Design review of the part built by this model. Coordinates are the model's own, in mm. Face numbers are marked on the shaded views. Coordinates: 2 decimals unless noted, no trailing zeros. Order: outer loops, then holes, each group sorted by start corner. A loop starts at its lowest first (then second) coordinate and runs counter-clockwise, first axis right, second up. Notation, with made-up numbers: M 87.5,57.5 L 135.5,57.5 A16 cw 135.5,75.5 Z; hole C -8.75,4.5 d7. An arc over 180 degrees is marked long. Answer in a Markdown table with one row per item.
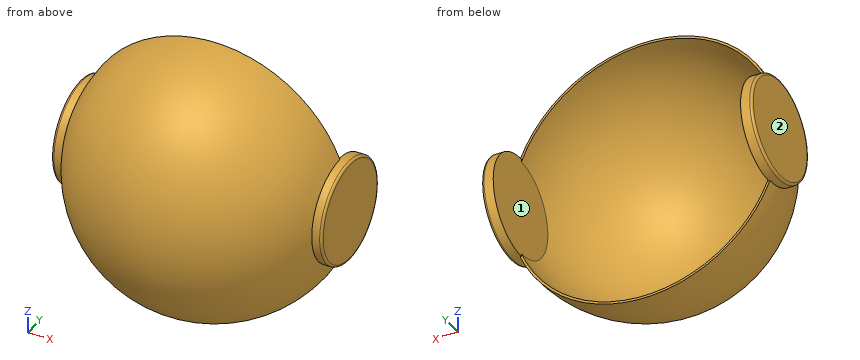
Autodesk Inventor part; units mm, degrees
ref_plane "Work Plane1" through (0, 0, 59) normal (0, 0, 1) x (1, 0, 0)
ref_plane "Work Plane2" through (-59, 0, 0) normal (1, 0, 0) x (0, 1, 0)
ref_plane "Work Plane3" through (59, 0, 0) normal (1, 0, 0) x (0, 1, 0)
sketch "Sketch1" plane through (0, 0, 0) normal (0, 0, 1) x (1, 0, 0)
  arc A0 (-59, 0) -> (59, 0) centre (0, 0) ccw
  arc A1 (-58, 0) -> (58, 0) centre (0, 0) ccw
  line L0 (-59, 0) -> (59, 0)
  dimension "d0" = 118
  dimension "d1" = 116
revolve "Revolution1" add sketch "Sketch1" angle 360 about axis through (-59, 0, 0) along (1, 0, 0) contours L0 A1 A0
ref_plane "Work Plane1" through (0, 0, 59) normal (0, 0, 1) x (1, 0, 0)
sketch "Sketch2" plane through (0, 0, 59) normal (0, 0, 1) x (1, 0, 0)
  circle A0 centre (0, 0) radius 59
  line L0 (-59, 0) -> (59, 0)
extrude "Extrusion1" cut sketch "Sketch2" against normal through all contours L0 A0 picked at (13.5288, 25.207)
ref_plane "Work Plane2" through (-59, 0, 0) normal (1, 0, 0) x (0, 1, 0)
sketch "Sketch3" plane through (-59, 0, 0) normal (1, 0, 0) x (0, 1, 0)
  circle A0 centre (0, 0) radius 22.5
  dimension "d5" = 45
extrude "Extrusion2" add sketch "Sketch3" along normal blind 5
fillet "Fillet1" radius 1 1 edges at (-59, -22.5, 0)
ref_plane "Work Plane3" through (59, 0, 0) normal (1, 0, 0) x (0, 1, 0)
sketch "Sketch4" plane through (59, 0, 0) normal (1, 0, 0) x (0, 1, 0)
  circle A0 centre (0, 0) radius 22.5
  point P0 (0, 22.5)
extrude "Extrusion3" add sketch "Sketch4" against normal blind 5
fillet "Fillet2" radius 1 1 edges at (59, -22.5, 0)
properties part number "Head"
(1) Draft analysis for pull direction Z (two halves, no side actions). For the marked faces 1 and 2, state which applies: pulls with the +Z half, pulls with the -Z half, needs draft (parallel to the pull), parting line crosses it, or undercut.
Return value:
| item | result |
|---|---|
| face 1 | undercut |
| face 2 | needs draft |
(2) For line 1 along X through (y, z) = (9, -17.5); line 2 along X through (y, z) = (-49, 4); line 3 along Z through (x, y) = (28.5, -21), list the stretches that pass through material, from the lowest coordinate up. Write a range as from..to.
Return value:
| item | result |
|---|---|
| line 1 | x = -59..-54, 54..59 |
| line 2 | x = -32.62..-30.77, 30.77..32.62 |
| line 3 | z = -47.2..-45.94, 45.94..47.2 |
(3) Add section A-A, the plane z = 0. Give the boundary of the cut face in (x, y).
Return value:
| item | result |
|---|---|
| outline | M -59,-21.5 A1 ccw -58,-22.5 L -54.54,-22.5 A59 ccw 54.54,-22.5 L 58,-22.5 A1 ccw 59,-21.5 L 59,21.5 A1 ccw 58,22.5 L 54,22.5 L 54,-21.17 A58 cw -54,-21.17 L -54,22.5 L -58,22.5 A1 ccw -59,21.5 Z |
(4) Add section D-D, the plane z = -38.5. Give the boundary of the cut face in (x, y).
Return value:
| item | result |
|---|---|
| outline | M -44.71,0 A44.71 ccw 44.71,0 L 43.38,0 A43.38 cw -43.38,0 Z |
(5) Insertion check: pin 1 Ø2 at (x, z) = (-16.5, 4.5) entering from +Y; pin 2 Ø10 at (x, y) = (-13.5, -47.5) entering from -Z; pin 3 Ø4 at (x, z) = (-35, 7) entering from -Y; pin 4 Ø1.5 at (y, z) = (-21.5, -3) entering from -X. Each pin has a flat end and moves straight along its axis. Give the tip position at first contact, or say it passes through.
Return value:
| item | result |
|---|---|
| pin 1 | stops at y = -55.1 |
| pin 2 | stops at z = -38.88 |
| pin 3 | stops at y = -48.43 |
| pin 4 | stops at x = -59 |
(6) Add section B-B, the plane x = 10. Give the boundary of the cut face in (y, z), and give its area (3 significant figures).
Return value:
| item | result |
|---|---|
| outline | M 0,-58.15 L 0,-57.13 A57.13 cw 0,57.13 L 0,58.15 A58.15 ccw Z |
| area | 184 mm2 |
(7) Add section C-C, the plane y = -43.5. Give the boundary of the cut face in (x, z), and give its area (3 significant figures).
Return value:
| item | result |
|---|---|
| outline | C 0,0 d79.72; hole C 0,0 d76.73 |
| area | 368 mm2 |
